Part model, mm, in its own coordinate system. A direction names the side the tool comes from. Round coordinates to 2 decimals unless told otherwise and drop trailing zeros. Loops run counter-clockwise (first coordinate to the right, second up) from the corner with the lowest first, then second, coordinate; pieces in that order, holes last. Notation, with made-up numbers: M 22.25,-32 L 46.25,-32 A29 ccw 46.25,-12 Z; hole C 16,9.25 d1. An arc over 180 degrees is marked long. Put each result on its own line as item: value. Start each with the question number.
1) Slice it at C-C on x = -18. Give the cut face in (y, z).
2) Which spindle directions (+Z, -Z, +X, -X, +Y, -Y) get a long thin tool onto all of the face, cutting with end or side? Do faces 5 (the flat face through (-1, 42, 27)), 6 (the cylindrical face through (-52.534, 2.958, 52.113)), 7 (the cylindrical face through (-21.983, 54.07, -0.855)). Say none if no direction does.
3) Pull direction Z, two halves, no side cores. Call faces 1 (the cylindrical face through (-7.283, 2.958, 54.516)), 2 (the cylindrical face through (-1.11, 57.48, 31.98)), 3 (the flat face through (1, 29, -32)), 4 (the flat face through (-1, 45, -25)): +Z half, -Z half, draft (parallel to the pull), parting line (faces both ways), or undercut.
4) Slice it at B-B on z = 20. Give the cut face in (x, y), then the cut area to 3 significant figures.
5) Slice it at A-A on x = 0. Give the cut face in (y, z), then the cut area to 4 significant figures.
6) Slice it at D-D on y = 13.5. Give the cut face in (x, z).
7) Drop flat-ended pins along their axis: pin 1 Ø1 at (y, z) = (15, 1.5) entering from +X; pin 2 Ø14.5 at (x, y) = (26.5, 37) entering from +Z; pin 3 Ø2 at (x, z) = (85.5, 31) entering from +Y; pin 4 Ø17.5 at (x, z) = (56, -32) entering from -Y. Give the stop position or say it passes through.
8) Probe line 1 along X through (y, z) = (43.25, 0); line 2 along X through (y, z) = (25, 46); line 3 along Z through (x, y) = (0, 16). List the from-to ranges inside material, lowest first.
```python
from build123d import *

# Parameters (mm, degrees)
BOSS_EXTRUDE1_DEPTH = 6
SKETCH2_R           = 5.5
CUT_EXTRUDE1_DEPTH  = 6
SKETCH3_R           = 50
BOSS_EXTRUDE2_DEPTH = 50
SKETCH4_R           = 37.5
BOSS_EXTRUDE3_DEPTH = 26
SKETCH5_R           = 32
BOSS_EXTRUDE4_DEPTH = 3
FILLET2_R           = 6
FILLET3_R           = 6
CUT_EXTRUDE2_START  = -27
CUT_EXTRUDE2_DEPTH  = 27
CUT_EXTRUDE3_DEPTH  = 10
SKETCH12_R          = 33
CUT_EXTRUDE9_DEPTH  = 29
SKETCH21_R          = 16
CUT_EXTRUDE16_DEPTH = 35
SKETCH22_R          = 45
CUT_EXTRUDE18_DEPTH = 21
SKETCH34_R          = 45
SKETCH34_R_2        = 25
CUT_EXTRUDE25_DEPTH = 8
CUT_EXTRUDE26_DEPTH = 13


with BuildPart() as part:
    # Sketch1 → Boss-Extrude1 (new body)
    with BuildSketch(Plane(origin=(0, 0, 0), x_dir=(1, 0, 0), z_dir=(0, 1, 0))):
        with BuildLine():
            ThreePointArc((21.211789327, -50.745048956), (28.860136885, -67.581936782), (43.965179902, -56.913493246))
            ThreePointArc((43.965179902, -56.913493246), (104.875389558, -29.654145663), (62.597817721, 21.976587342))
            ThreePointArc((62.597817721, 21.976587342), (62.107138398, 42.329707672), (44.037643352, 32.949749135))
            ThreePointArc((44.037643352, 32.949749135), (8.49481412, 54.340023308), (-31.880473469, 44.817802394))
            ThreePointArc((-31.880473469, 44.817802394), (-52.325901808, 52.325901808), (-44.817802394, 31.880473469))
            ThreePointArc((-44.817802394, 31.880473469), (-55, 0), (-44.817802394, -31.880473469))
            ThreePointArc((-44.817802394, -31.880473469), (-52.325901808, -52.325901808), (-31.880473469, -44.817802394))
            ThreePointArc((-31.880473469, -44.817802394), (-6.102316632, -54.660421986), (21.211789327, -50.745048956))
        make_face()
    extrude(amount=BOSS_EXTRUDE1_DEPTH)

    # Sketch2 → Cut-Extrude1 (cut)
    with BuildSketch(Plane(origin=(0, 6, 0), x_dir=(1, 0, 0), z_dir=(0, 1, 0))):
        with Locations(Location((56, 32, 0), (0, 0, 270))):
            Circle(SKETCH2_R)
        with Locations(Location((-43.840620434, 43.840620434, 0), (0, 0, 270))):
            Circle(SKETCH2_R)
        with Locations(Location((-43.840620434, -43.840620434, 0), (0, 0, 270))):
            Circle(SKETCH2_R)
        with Locations(Location((32, -56, 0), (0, 0, 270))):
            Circle(SKETCH2_R)
    extrude(amount=-CUT_EXTRUDE1_DEPTH, mode=Mode.SUBTRACT)

    # Sketch3 → Boss-Extrude2 (add)
    with BuildSketch(Plane(origin=(0, 6, 0), x_dir=(1, 0, 0), z_dir=(0, 1, 0))):
        with Locations(Location((0, 0, 0), (0, 0, 270))):
            Circle(SKETCH3_R)
    extrude(amount=BOSS_EXTRUDE2_DEPTH)

    # Sketch4 → Boss-Extrude3 (add)
    with BuildSketch(Plane(origin=(0, 6, 0), x_dir=(1, 0, 0), z_dir=(0, 1, 0))):
        with Locations((64, -20)):
            Circle(SKETCH4_R)
    extrude(amount=BOSS_EXTRUDE3_DEPTH)

    # Sketch5 → Boss-Extrude4 (add)
    with BuildSketch(Plane(origin=(0, 56, 0), x_dir=(1, 0, 0), z_dir=(0, 1, 0))):
        with Locations(Location((0, 0, 0), (0, 0, 270))):
            Circle(SKETCH5_R)
    extrude(amount=BOSS_EXTRUDE4_DEPTH)

    # Fillet2
    fillet2_edges = [part.edges().sort_by_distance(p)[0] for p in [
        (44.037643352, 3, -32.949749135),
    ]]
    fillet(fillet2_edges, radius=FILLET2_R)

    # Fillet3
    fillet3_edges = [part.edges().sort_by_distance(p)[0] for p in [
        (21.211789327, 3, 50.745048956),
        (-31.880473469, 3, 44.817802394),
        (-44.817802394, 3, 31.880473469),
        (-44.817802394, 3, -31.880473469),
        (-31.880473469, 3, -44.817802394),
        (62.597817721, 3, -21.976587342),
        (43.965179902, 3, 56.913493246),
    ]]
    fillet(fillet3_edges, radius=FILLET3_R)

    # Sketch6 → Cut-Extrude2 (cut)
    with BuildSketch(Plane(origin=(0, 59, 0), x_dir=(1, 0, 0), z_dir=(0, 1, 0)).offset(CUT_EXTRUDE2_START)):
        with BuildLine():
            Line((0, 25), (43.301270189, 25))
            ThreePointArc((43.301270189, 25), (0, 50), (-43.301270189, 25))
            Line((-43.301270189, 25), (0, 25))
        make_face()
    extrude(amount=CUT_EXTRUDE2_DEPTH, mode=Mode.SUBTRACT)

    # Sketch7 → Cut-Extrude3 (cut)
    with BuildSketch(Plane(origin=(0, 59, 0), x_dir=(1, 0, 0), z_dir=(0, 1, 0))):
        with BuildLine():
            ThreePointArc((20.545454545, 7.866657328), (-22, 0), (20.545454545, -7.866657328))
            ThreePointArc((20.545454545, -7.866657328), (30, 0), (20.545454545, 7.866657328))
        make_face()
    extrude(amount=-CUT_EXTRUDE3_DEPTH, mode=Mode.SUBTRACT)

    # Sketch12 → Cut-Extrude9 (cut)
    with BuildSketch(Plane.XZ):
        with Locations(Location((64, 20, 0), (0, 0, 270))):
            Circle(SKETCH12_R)
    extrude(amount=-CUT_EXTRUDE9_DEPTH, mode=Mode.SUBTRACT)

    # Sketch21 → Cut-Extrude16 (cut)
    with BuildSketch(Plane(origin=(0, 56, 0), x_dir=(1, 0, 0), z_dir=(0, 1, 0))):
        with Locations(Location((0, 0, 0), (0, 0, 270))):
            Circle(SKETCH21_R)
    extrude(amount=-CUT_EXTRUDE16_DEPTH, mode=Mode.SUBTRACT)

    # Sketch22 → Cut-Extrude18 (cut)
    with BuildSketch(Plane.XZ):
        Circle(SKETCH22_R)
    extrude(amount=-CUT_EXTRUDE18_DEPTH, mode=Mode.SUBTRACT)

    # Sketch34 → Cut-Extrude25 (cut)
    with BuildSketch(Plane(origin=(0, 21, 0), x_dir=(-1, 0, 0), z_dir=(0, -1, 0))):
        Circle(SKETCH34_R)
        with Locations(Location((0, 0, 0), (0, 0, 90))):
            Circle(SKETCH34_R_2, mode=Mode.SUBTRACT)
    extrude(amount=-CUT_EXTRUDE25_DEPTH, mode=Mode.SUBTRACT)

    # Sketch35 → Cut-Extrude26 (cut)
    with BuildSketch(Plane.XZ.offset(-29)):
        with BuildLine():
            Line((15, -20), (40.311288741, -20))
            ThreePointArc((40.311288741, -20), (0, 45), (-40.311288741, -20))
            Line((-40.311288741, -20), (-15, -20))
            ThreePointArc((-15, -20), (-13.588689929, 20.984458678), (24.386363636, 5.505022125))
            ThreePointArc((24.386363636, 5.505022125), (28, 0), (24.386363636, -5.505022125))
            ThreePointArc((24.386363636, -5.505022125), (20.984458678, -13.588689929), (15, -20))
        make_face()
    extrude(amount=-CUT_EXTRUDE26_DEPTH, mode=Mode.SUBTRACT)


solid = part.part
```
Recorded:
1. outline: M 0,-51.97 L 6,-51.97 L 6,-46.65 L 32,-46.65 L 32,-25 L 59,-25 L 59,-12.65 L 49,-12.65 L 49,12.65 L 59,12.65 L 59,26.46 L 56,26.46 L 56,46.65 L 6,46.65 L 6,51.97 L 0,51.97 L 0,41.24 L 42,41.24 L 42,17.35 L 21,17.35 L 21,-17.35 L 42,-17.35 L 42,-20 L 29,-20 L 29,-41.24 L 0,-41.24 Z
2. face 5: -Y
2. face 6: +Y, -Y
2. face 7: +Y
3. face 1: +Z half
3. face 2: parting line
3. face 3: undercut
3. face 4: -Z half
4. outline: M -51.23,0 L -40.31,0 L -40.31,42 L -15,42 L -15,21 L 15,21 L 15,42 L 40.31,42 L 40.31,29 L 97,29 L 97,0 L 106,0 L 106,6 L 101.5,6 L 101.5,32 L 45.83,32 L 45.83,56 L 24.98,56 L 24.98,59 L 9.17,59 L 9.17,49 L -9.17,49 L -9.17,59 L -24.98,59 L -24.98,56 L -45.83,56 L -45.83,6 L -51.23,6 Z
4. area: 2,540 mm2
5. outline: M 0,-55 L 6,-55 L 6,-50 L 32,-50 L 32,-25 L 59,-25 L 59,-22 L 49,-22 L 49,-16 L 21,-16 L 21,-25 L 29,-25 L 29,-45 L 0,-45 Z; M 0,45 L 42,45 L 42,25 L 21,25 L 21,16 L 49,16 L 49,22 L 59,22 L 59,32 L 56,32 L 56,50 L 6,50 L 6,55 L 0,55 Z
5. area: 1,425 mm2
6. outline: M 31.55,38.79 A50 ccw long 48.02,-13.93 A37.5 ccw long Z; hole M 32.81,30.79 A45 ccw long 44.51,-6.63 A33 ccw long Z
7. pin 1: stops at x = 96.9
7. pin 2: stops at z = 46.15
7. pin 3: stops at y = 32
7. pin 4: stops at y = 0
8. line 1: x = -50 to -16, 16 to 50
8. line 2: x = -19.6 to 19.6, 36.98 to 43.68, 84.32 to 91.02
8. line 3: z = -50 to -45, 45 to 50
